Here's how the part is built. I have some questions about the finished solid (model axes, mm). Coordinates: 2 decimals unless noted, no trailing zeros. Write each loop counter-clockwise with the first axis right and the second up, starting at its lowest first coordinate (ties: lowest second). Pieces come first, ordered by that corner, then holes.
```python
from build123d import *

# Parameters (mm, degrees)
SKETCH1_R      = 2.38125
EXTRUDE1_DEPTH = 4.7625
FILLET1_R      = 0.79375
CHAMFER1_SIZE  = 0.79375


with BuildPart() as part:
    # Sketch1 → Extrude1 (new, symmetric)
    with BuildSketch(Plane.XY):
        with Locations(Location((0, 0, 0), (0, 0, 180))):
            Circle(SKETCH1_R)
    extrude(amount=EXTRUDE1_DEPTH, both=True)

    # Fillet1
    fillet1_edges = [part.edges().sort_by_distance(p)[0] for p in [
        (2.38125, 0, 4.7625),
    ]]
    fillet(fillet1_edges, radius=FILLET1_R)

    # Chamfer1
    chamfer1_edges = [part.edges().sort_by_distance(p)[0] for p in [
        (2.38125, 0, -4.7625),
    ]]
    chamfer(chamfer1_edges, length=CHAMFER1_SIZE)


solid = part.part
```
1) Will these pins go through, and if not, where does the flat tip stop? pin 1 (1 mm diameter, centred on x = -1.5, z = -3.5, fed in from -Y); pin 2 (1.5 mm diameter, centred on x = -1, z = 2.5, fed in from -Y).
Values follow:
pin 1: stops at y = -2.16
pin 2: stops at y = -2.37
2) I need wall thicknesses on probe 1 along X at (y, z) = (0.6, 0.25); probe 2 along Y at (x, z) = (1.35, -4); probe 3 along X at (y, z) = (0.85, 3). Which ranges of each line are inside material? Lowest first, please.
Values follow:
probe 1: x = -2.3 to 2.3
probe 2: y = -1.92 to 1.92
probe 3: x = -2.22 to 2.22
3) Imagine slicing it at C-C on z = -2.5. Please give me the cut outline in (x, y), then the cut area to 3 significant figures.
Values follow:
outline: circle Ø4.76 at (0, 0)
area: 17.8 mm2
4) Imagine slicing it at A-A on y = 0. Please give me the cut outline in (x, z), then the cut area to 3 significant figures.
Values follow:
outline: (-2.38, -3.97) - (-1.59, -4.76) - (1.59, -4.76) - (2.38, -3.97) - (2.38, 3.97) arc R0.79 ccw to (1.59, 4.76) - (-1.59, 4.76) arc R0.79 ccw to (-2.38, 3.97) - close
area: 44.5 mm2
